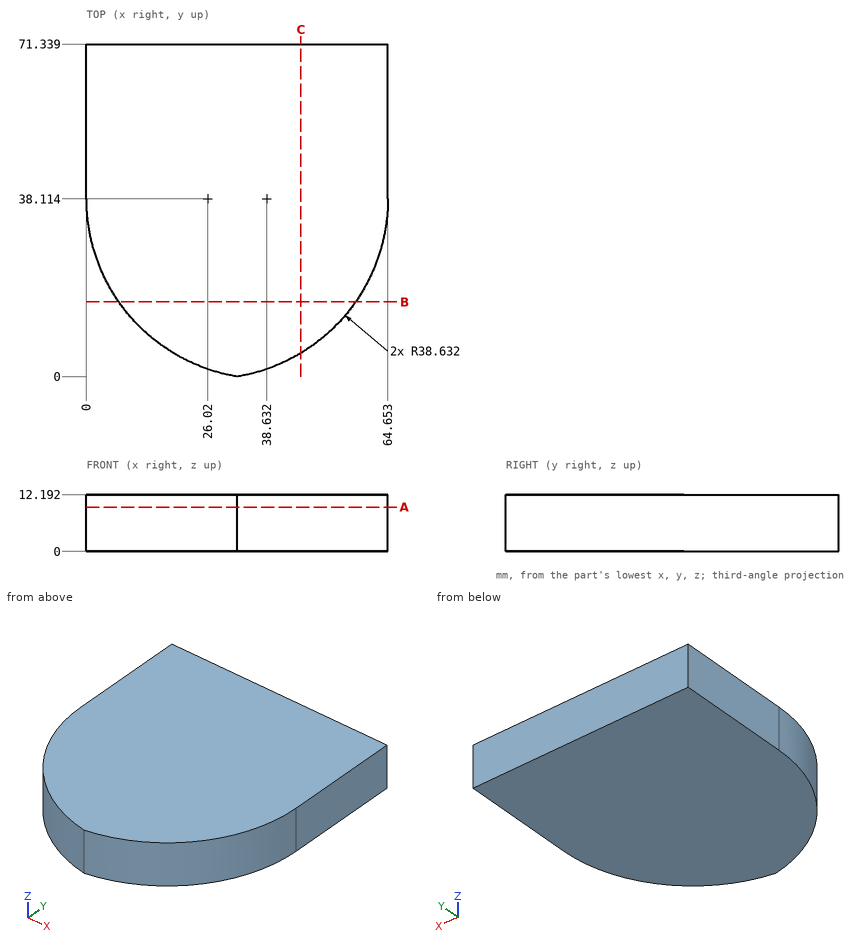
Design review of the part shown in the three views and the two pictorial views. Dimensions are in mm from the part's minimum x, y and z. Give positions to 0.01 mm unless a question says otherwise; leave off trailing zeros. Loops run counter-clockwise (first coordinate to the right, second up) from the corner with the lowest first, then second, coordinate; pieces in that order, holes last. Notation, with made-up numbers: M 22.5,17.5 L 68.5,17.5 A19 cw 68.5,31.5 Z; hole C 45.25,-20 d11. An arc over 180 degrees is marked long. Answer as a JSON object with one key per item and string values. Group by question number.
Q1. Insertion check: P1, Ø4, axis at y = 22.5, z = 3, coming from the +X side (1 decimal); P2, Ø3, axis at x = 36.5, z = 8, coming from the -Y side; P3, Ø1, axis at y = 31, z = 6, coming from the -X side. Each pin has a flat end and moves straight along its axis. Give the tip position at first contact, or say it passes through.
Q2. Add section C-C on x = 46. Give the boundary of the cut face in (y, z), and give its area (3 significant figures).
Q3. Add section A-A on z = 9.5. Give the boundary of the cut face in (x, y) (1 decimal).
Q4. For probe 1 along X at (y, z) = (15.5, 6.5); probe 2 along X at (y, z) = (17, 10); probe 3 along Y at (x, z) = (7.5, 11.5), list the stretches that pass through material, from the lowest coordinate up. Write a range as [from, to].
Q5. Add section B-B on y = 16. Give the boundary of the cut face in (x, z) (1 decimal).
Checked values:
{
 "1": {"P1": "x = 62.2", "P2": "y = 0.54", "P3": "x = 0.57"},
 "2": {"outline": "M 5.05,0 L 71.34,0 L 71.34,12.19 L 5.05,12.19 Z", "area": "808 mm²"},
 "3": {"outline": "M 0,38.1 A38.6 ccw 32.3,0 A38.6 ccw 64.7,38.1 L 64.7,71.3 L 0,71.3 Z"},
 "4": {"probe 1": "[7.31, 57.34]", "probe 2": "[6.28, 58.37]", "probe 3": "[15.24, 71.34]"},
 "5": {"outline": "M 7,0 L 57.7,0 L 57.7,12.2 L 7,12.2 Z"}
}
